Autodesk Inventor part; units mm, degrees
ref_plane "YZ Plane" through (0, 0, 0) normal (1, 0, 0) x (0, 1, 0)
ref_plane "XZ Plane" through (0, 0, 0) normal (0, 1, 0) x (-1, 0, 0)
ref_plane "XY Plane" through (0, 0, 0) normal (0, 0, 1) x (1, 0, 0)
sketch "Sketch1" plane through (0, 0, 0) normal (0, 0, 1) x (1, 0, 0)
  line L0 (15.875, -34.925) -> (-15.875, -34.925)
  line L1 (-15.875, -34.925) -> (-15.875, 34.925)
  line L2 (-15.875, 34.925) -> (15.875, 34.925)
  line L3 (15.875, 34.925) -> (15.875, -34.925)
  line L4 (15.875, -34.925) -> (-15.875, 34.925) construction
  line L5 (-15.875, -34.925) -> (15.875, 34.925) construction
  point P0 (0, 0)
  dimension "d0" = 31.75
  dimension "d1" = 69.85
extrude "Extrusion1" add sketch "Sketch1" along normal blind 38.1
sketch "Sketch2" plane through (0, 0, 38.1) normal (0, 0, 1) x (1, 0, 0)
  line L0 (9.525, -28.575) -> (-15.875, -28.575)
  line L1 (-15.875, -28.575) -> (-15.875, -3.175)
  line L2 (-15.875, -3.175) -> (9.525, -3.175)
  line L3 (9.525, -3.175) -> (9.525, -28.575)
  line L4 (-15.875, -34.925) -> (15.875, -34.925)
  line L5 (15.875, -34.925) -> (15.875, 34.925)
  line L6 (-15.875, 34.925) -> (-15.875, -34.925)
  point P0 (0, 0)
  dimension "d4" = 6.35
  dimension "d5" = 6.35
  dimension "d6" = 25.4
  dimension "d7" = 25.4
extrude "Extrusion2" cut sketch "Sketch2" against normal through all
sketch "Sketch3" plane through (15.875, -34.925, 0) normal (1, 0, 0) x (0, 0, -1)
  line L0 (-38.1, 69.85) -> (-38.1, 31.75)
  line L1 (-38.1, 50.8) -> (-15.875, 69.85)
  line L2 (0, 69.85) -> (-38.1, 69.85)
  line L3 (-38.1, 50.8) -> (-38.1, 69.85)
  line L4 (-38.1, 69.85) -> (-15.875, 69.85)
  line L5 (0, 0) -> (0, 69.85)
  arc A0 (-15.875, 69.85) -> (0, 69.85) centre (-7.9375, 93.9779) ccw
  line L6 (0, 69.85) -> (-38.1, 69.85)
  line L7 (-15.875, 69.85) -> (0, 69.85)
  point P0 (0, 34.925)
  dimension "d10" = 15.875
  dimension "d11" = 19.05
  dimension "d23" = 25.4
extrude "Extrusion3" cut sketch "Sketch3" against normal through all
sketch "Sketch4" plane through (-15.875, -34.925, 0) normal (0, -1, 0) x (1, 0, 0)
  circle A0 centre (12.7, 25.4) radius 3.3734
  line L0 (0, 0) -> (0, 38.1)
  line L1 (0, 38.1) -> (31.75, 38.1)
  point P0 (15.875, 0)
  dimension "d14" = 12.7
  dimension "d15" = 12.7
  dimension "d16" = 6.7469
extrude "Extrusion4" cut sketch "Sketch4" against normal through all
ref_plane "Work Plane1" through (-15.875, 9.525, 38.1) normal (0, -1, 0) x (1, 0, 0)
sketch "Sketch5" plane through (-15.875, 9.525, 38.1) normal (0, -1, 0) x (1, 0, 0)
  circle A0 centre (12.7, -12.7) radius 3.3734
  line L0 (7.1437, -9.4921) -> (12.7, -6.2842)
  line L1 (12.7, -6.2842) -> (18.2563, -9.4921)
  line L2 (18.2563, -9.4921) -> (18.2562, -15.9079)
  line L3 (18.2562, -15.9079) -> (12.7, -19.1158)
  line L4 (12.7, -19.1158) -> (7.1437, -15.9079)
  line L5 (7.1437, -15.9079) -> (7.1437, -9.4921)
  point P0 (15.875, -38.1)
  dimension "d20" = 11.1125
extrude "Extrusion5" cut sketch "Sketch5" against normal blind 38.1 contours A0 | L0 L1 L2 L3 L4 L5
fillet "Fillet1" radius 3.175 1 edges at (0, 34.925, 15.875)
chamfer "Chamfer1" distance 3.175 angle 45 1 edges at (0, 34.925, 0)
fillet "Fillet2" radius 3.175 1 edges at (0, 34.1233, 3.0721)
sketch "Sketch6" plane through (15.875, -34.925, 38.1) normal (1, 0, 0) x (0, 0, -1)
  line L0 (25.4, 0) -> (38.1, 63.5)
  line L1 (38.1, 63.5) -> (38.1, 0)
  line L2 (38.1, 0) -> (25.4, 0)
  line L3 (38.1, 0) -> (0, 0)
  line L4 (38.1, 0) -> (38.1, 66.675)
  line L5 (-4.7298, -21.134) -> (20.7966, 106.498)
  line L6 (20.7966, 106.498) -> (-6.997, 112.0567)
  line L7 (-6.997, 112.0567) -> (-32.5234, -15.5753)
  line L8 (-32.5234, -15.5753) -> (-4.7298, -21.134)
  point P0 (38.1, 34.925)
  dimension "d29" = 63.5
  dimension "d30" = 12.7
  dimension "d33" = 25.4
extrude "Extrusion6" cut sketch "Sketch6" against normal through all
properties part number "IntakeStop"
For this review, take the finished solid that the model builds, in its own axes (mm). A direction names the side the tool comes from. Coordinates: 2 decimals unless noted, no trailing zeros. Loops run counter-clockwise (first coordinate to the right, second up) from the corner with the lowest first, then second, coordinate; pieces in that order, holes last. Notation, with made-up numbers: (32, 85) - (63, 85) arc R22 cw to (63, 109) - close; hole circle Ø2 at (59.5, -26.5). An arc over 180 degrees is marked (long way). Return JSON: item names as keys, results as strings.
Item 1: For line 1 (Y direction, x = -8.5, z = 25) (3 decimals); line 2 (Y direction, x = 6, z = 17) (3 decimals); line 3 (Y direction, x = -8, z = 32.5) (3 decimals), list the stretches that pass through material, from the lowest coordinate up.
Determined:
{"line 1": "y = -34.925 to -28.575, -3.175 to 9.525", "line 2": "y = -34.925 to -28.575, -3.175 to 33.95", "line 3": "y = -34.925 to -28.575"}
Item 2: For faces 1 (the flat face through (9.525, -16, 22)), 2 (the flat face through (-2, 9.525, 22)), 3 (the flat face through (0, -34.925, 28)), list the 3-axis set-ups (+Z, -Z, +X, -X, +Y, -Y) from which the entire face can be reached by the end or side of a thin tool; tool diameter is ignored.
Determined:
{"face 1": "+Z, -Z, -X", "face 2": "+Y", "face 3": "+Z, -Z, +X, -X, -Y"}
Item 3: Mouldability with a two-part tool opening along Z and no side actions: class faces 4 (the cylindrical face through (0.22, 33.83, 3.09)), 5 (the flat face through (0, 30, 0)), 6 (the flat face through (3.75, 2.79, 31.06)) as pulls with the +Z half, pulls with the -Z half, needs draft (parallel to the pull), parting line crosses it, or undercut.
Determined:
{"face 4": "undercut", "face 5": "pulls with the -Z half", "face 6": "pulls with the +Z half"}
Item 4: Take a section at A-A (z = 25.4). Give the boundary of the cut face in (x, y) (3 decimals).
Determined:
{"outline": "(-15.875, -34.925) - (-6.548, -34.925) - (-6.548, -28.575) - (-15.875, -28.575) - close; (-15.875, -3.175) - (-6.548, -3.175) - (-6.548, 9.525) - (-8.731, 9.525) - (-8.731, 26.761) - (-15.875, 26.761) - close; (0.198, -34.925) - (15.875, -34.925) - (15.875, 26.761) - (2.381, 26.761) - (2.381, 9.525) - (0.198, 9.525) - (0.198, -3.175) - (9.525, -3.175) - (9.525, -28.575) - (0.198, -28.575) - close"}
Item 5: Take a section at C-C (y = 1). Give the boundary of the cut face in (x, z) (3 decimals), then the cut area to 3 significant figures.
Determined:
{"outline": "(-15.875, 5.515) - (15.875, 5.515) - (15.875, 31.418) - (-15.875, 31.418) - close; hole circle Ø6.747 at (-3.175, 25.4)", "area": "787 mm2"}
Item 6: Insertion check: pin 1 (8 mm diameter, centred on x = -3.5, y = -0.5, fed in from -Z) (3 decimals); pin 2 (10 mm diameter, centred on x = 4, y = -3, fed in from -Z) (3 decimals); pin 3 (1 mm diameter, centred on x = 10, y = 17.5, fed in from +Z). Each pin has a flat end and moves straight along its axis. Give the tip position at first contact, or say it passes through.
Determined:
{"pin 1": "stops at z = 5.015", "pin 2": "stops at z = 5.315", "pin 3": "stops at z = 28.22"}
Item 7: Take a section at B-B (x = -4.5). State how many separate pieces and enclosed holes the cut face has, then the cut area to 3 significant figures.
Determined:
{"separate pieces": "4", "enclosed holes": "0", "area": "815 mm2"}
